Here's how the part is built. I have some questions about the finished solid (model axes, mm). A direction names the side the tool comes from. Give positions to 0.01 mm unless a question says otherwise; leave off trailing zeros. Loops run counter-clockwise (first coordinate to the right, second up) from the corner with the lowest first, then second, coordinate; pieces in that order, holes last. Notation, with made-up numbers: (58, 28.25) -> (108, 28.25) arc R10 ccw to (108, 33.25) -> close; hole circle Ø7 at (-26.5, 80.25). An arc over 180 degrees is marked (long way). Answer in a Markdown table with one row per item. Add a question column.
Item 1: For P1, Ø1.5, axis at y = 25.5, z = -9, coming from the +X side; P2, Ø8, axis at x = -19, z = -1, coming from the +Y side; P3, Ø2.5, axis at x = 20.5, z = 20.5, coming from the +Y side, each with a flat end and sliding along its axis, tell me the tip position at first contact or that it passes through.
Item 2: We'd pull the mould along Z, two halves only. Please class faces 1 (the face through (-27.5, 26, 17)), 2 (the face through (-11.5, 26, 0)): released by +Z, released by -Z, zero draft, split by the parting line, or undercut.
Item 3: Which directions (+Z, -Z, +X, -X, +Y, -Y) give clear straight access to the entire face, cutting with the end or side of a thin tool? Please do faces 3 (the face through (-12, 26, -9)), 4 (the face through (-27.5, 26, -18)), 5 (the face through (-22.5, 25.1, 19.9)), 6 (the face through (27.5, 26, 0)).
Item 4: If I drill on line 1 (Z direction, x = -10, y = 22.75); line 2 (Z direction, x = 8.5, y = 23.5); line 3 (Z direction, x = -20, y = 24), over which ranges is the centre line in solid material (lowest first)?
Item 5: If we section it at A-A (y = 18): Write out the boundary of the cut face in (x, z), then the cut area to 3 significant figures.
Item 6: If we section it at C-C (z = -21): Write out the boundary of the cut face in (x, y).
Item 7: If we section it at D-D (y = 26.5): Give the number of separate pieces and of enclosed holes in the cut face, then the cut area to 3 significant figures.
Item 8: If we section it at B-B (x = -10): Write out the boundary of the cut face in (y, z), then the cut area to 3 significant figures.
Autodesk Inventor part; units mm, degrees
ref_plane "YZ Plane" through (0, 0, 0) normal (1, 0, 0) x (0, 1, 0)
ref_plane "XZ Plane" through (0, 0, 0) normal (0, 1, 0) x (-1, 0, 0)
ref_plane "XY Plane" through (0, 0, 0) normal (0, 0, 1) x (1, 0, 0)
sketch "Sketch1" plane through (0, 0, 0) normal (0, 1, 0) x (-1, 0, 0)
  line L0 (30, 30) -> (-30, 30)
  line L1 (-30, 30) -> (-30, -30)
  line L2 (-30, -30) -> (30, -30)
  line L3 (30, -30) -> (30, 30)
  line L4 (30, 30) -> (-30, -30) construction
  line L5 (-30, 30) -> (30, -30) construction
  point P0 (0, 0)
  dimension "d0" = 60
  dimension "d1" = 60
extrude "Extrusion1" add sketch "Sketch1" along normal blind 22.5
sketch "Sketch2" plane through (0, 22.5, 0) normal (0, 1, 0) x (1, 0, 0)
  line L0 (-27.5, -27.5) -> (27.5, -27.5)
  line L1 (27.5, -27.5) -> (27.5, 27.5)
  line L2 (27.5, 27.5) -> (-27.5, 27.5)
  line L3 (-27.5, 27.5) -> (-27.5, -27.5)
  line L4 (-27.5, -27.5) -> (27.5, 27.5) construction
  line L5 (27.5, -27.5) -> (-27.5, 27.5) construction
  line L6 (30, 30) -> (-30, 30)
  line L7 (-30, 30) -> (-30, -30)
  point P0 (0, 0)
  dimension "d4" = 2.5
  dimension "d5" = 2.5
extrude "Extrusion2" add sketch "Sketch2" along normal blind 7.5
sketch "Sketch5" plane through (0, 30, 0) normal (0, 1, 0) x (1, 0, 0)
  point P0 (0, 0)
sketch "Sketch6" plane through (0, 30, 0) normal (0, 1, 0) x (1, 0, 0)
  circle A0 centre (20, 22.5) radius 2.5
  circle A1 centre (-20, 22.5) radius 2.5
  line L0 (-30, -30) -> (30, -30)
  line L1 (30, -30) -> (30, 30)
  line L2 (-30, 30) -> (-30, -30)
  circle A2 centre (20, -20) radius 2.5
  circle A3 centre (-20, -20) radius 2.5
  line L3 (-27.5, -27.5) -> (27.5, -27.5)
  line L4 (27.5, 27.5) -> (-27.5, 27.5)
  circle A4 centre (-10, -20) radius 2.5
  circle A5 centre (-10, 22.5) radius 2.5
  point P0 (0, 0)
  dimension "d15" = 5
  dimension "d16" = 52.5
  dimension "d17" = 52.5
  dimension "d18" = 10
  dimension "d19" = 10
  dimension "d20" = 5
  dimension "d21" = 5
  dimension "d22" = 10
  dimension "d23" = 10
  dimension "d24" = 10
  dimension "d25" = 10
  dimension "d26" = 5
  dimension "d27" = 55
  dimension "d28" = 57.5
  dimension "d66" = 5
  dimension "d67" = 5
  dimension "d68" = 40
  dimension "d69" = 40
extrude "Extrusion5" cut sketch "Sketch6" against normal blind 10
sketch "Sketch7" plane through (0, 30, 0) normal (0, 1, 0) x (1, 0, 0)
  arc A0 (8.5, -12.5) -> (8.5, 12.5) centre (8.5, 0) ccw
  line L0 (30, -30) -> (30, 30)
  line L1 (8.5, 0) -> (8.5, 12.5)
  line L2 (8.5, 0) -> (8.5, -12.5)
  point P0 (0, 0)
  dimension "d32" = 21.5
extrude "Extrusion6" cut sketch "Sketch7" against normal blind 10
sketch "Sketch8" plane through (0, 30, 0) normal (0, 1, 0) x (1, 0, 0)
  line L0 (-4, -17.5) -> (6, -17.5)
  line L1 (8.5, -15) -> (8.5, 15)
  line L2 (6, 17.5) -> (-4, 17.5)
  line L3 (-6.5, 15) -> (-6.5, -15)
  line L4 (-6.5, -17.5) -> (8.5, 17.5) construction
  line L5 (8.5, -17.5) -> (-6.5, 17.5) construction
  line L6 (30, -30) -> (30, 30)
  line L7 (8.5, -12.5) -> (8.5, 12.5)
  arc A0 (8.5, 12.5) -> (8.5, -12.5) centre (8.5, 0) ccw
  arc A1 (-4, 17.5) -> (-6.5, 15) centre (-4, 15) ccw
  arc A2 (8.5, 15) -> (6, 17.5) centre (6, 15) ccw
  arc A3 (-6.5, -15) -> (-4, -17.5) centre (-4, -15) ccw
  arc A4 (6, -17.5) -> (8.5, -15) centre (6, -15) ccw
  point P0 (0, 0)
  point P1 (1, 0)
  dimension "d35" = 35
  dimension "d37" = 21.5
extrude "Extrusion7" cut sketch "Sketch8" against normal blind 5
sketch "Sketch9" plane through (0, 25, 0) normal (0, 1, 0) x (1, 0, 0)
  line L0 (8.5, -12.5) -> (8.5, 12.5)
  arc A0 (8.5, 12.5) -> (8.5, -12.5) centre (8.5, 0) ccw
  line L1 (8.5, -12.5) -> (8.5, -15)
  line L2 (8.5, 15) -> (8.5, 12.5)
  line L3 (8.5, -12.5) -> (8.5, 12.5)
  point P0 (0, 0)
extrude "Extrusion8" cut sketch "Sketch9" against normal blind 5
sketch "Sketch11" plane through (8.5, 20, 0) normal (0, 1, 0) x (1, 0, 0)
  circle A0 centre (0, 0) radius 2.5
  line L0 (21.5, -30) -> (21.5, 30)
  point P0 (-8.5, 0)
  dimension "d55" = 21.5
  dimension "d56" = 5
extrude "Extrusion10" cut sketch "Sketch11" against normal blind 10
sketch "Sketch12" plane through (0, 30, 0) normal (0, 1, 0) x (1, 0, 0)
  line L0 (-27.5, -27.5) -> (-27.5, 27.5)
  line L1 (-27.5, 0) -> (-19.0189, 0)
  line L2 (-27.5, 10) -> (-27.5, -10)
  line L3 (-11.5, -7.5) -> (-11.5, 7.5)
  line L4 (-14, 10) -> (-27.5, 10)
  line L5 (-14, -10) -> (-27.5, -10)
  line L6 (30, -30) -> (30, 30)
  arc A0 (-11.5, 7.5) -> (-14, 10) centre (-14, 7.5) ccw
  arc A1 (-14, -10) -> (-11.5, -7.5) centre (-14, -7.5) ccw
  point P0 (0, 0)
  dimension "d59" = 20
  dimension "d60" = 10
  dimension "d61" = 41.5
extrude "Extrusion11" cut sketch "Sketch12" against normal blind 7.5
sketch "Sketch13" plane through (0, 30, 0) normal (0, 1, 0) x (1, 0, 0)
  point P0 (0, 0)
sketch "Sketch14" plane through (0, 22.5, 0) normal (0, 1, 0) x (1, 0, 0)
  circle A0 centre (-21.5, 0) radius 5
  line L0 (30, -30) -> (30, 30)
  point P0 (0, 0)
  dimension "d70" = 10
  dimension "d71" = 51.5
extrude "Extrusion12" cut sketch "Sketch14" against normal blind 10
fillet "Fillet1" radius 2.5 1 edges at (-27.5, 26.25, -27.5)
fillet "Fillet2" radius 2.5 1 edges at (-27.5, 26.25, 27.5)
fillet "Fillet3" radius 2.5 1 edges at (27.5, 26.25, 27.5)
fillet "Fillet4" radius 2.5 1 edges at (27.5, 26.25, -27.5)
properties part number "Exercise1"
Recorded:
| question | item | result |
|---|---|---|
| 1 | P1 | stops at x = 27.5 |
| 1 | P2 | stops at y = 22.5 |
| 1 | P3 | stops at y = 20 |
| 2 | face 1 | zero draft |
| 2 | face 2 | undercut |
| 3 | face 3 | -X, +Y |
| 3 | face 4 | +Z, -Z, -X, +Y |
| 3 | face 5 | +Y |
| 3 | face 6 | +Z, -Z, +X, +Y |
| 4 | line 1 | z = -27.5 to -25, -20 to 17.5, 22.5 to 27.5 |
| 4 | line 2 | z = -27.5 to -12.5, 12.5 to 27.5 |
| 4 | line 3 | z = -27.5 to -25, -20 to -10, 10 to 17.5, 22.5 to 27.5 |
| 5 | outline | (-30, -30) -> (30, -30) -> (30, 30) -> (-30, 30) -> close; hole circle Ø10 at (-21.5, 0); hole circle Ø5 at (8.5, 0) |
| 5 | area | 3,500 mm^2 |
| 6 | outline | (-30, 0) -> (30, 0) -> (30, 22.5) -> (27.5, 22.5) -> (27.5, 30) -> (22, 30) -> (22, 20) -> (18, 20) -> (18, 30) -> (-8, 30) -> (-8, 20) -> (-12, 20) -> (-12, 30) -> (-18, 30) -> (-18, 20) -> (-22, 20) -> (-22, 30) -> (-27.5, 30) -> (-27.5, 22.5) -> (-30, 22.5) -> close |
| 7 | separate pieces | 1 |
| 7 | enclosed holes | 7 |
| 7 | area | 1,820 mm^2 |
| 8 | outline | (0, -30) -> (22.5, -30) -> (22.5, -27.5) -> (30, -27.5) -> (30, -25) -> (20, -25) -> (20, -20) -> (30, -20) -> (30, 17.5) -> (20, 17.5) -> (20, 22.5) -> (30, 22.5) -> (30, 27.5) -> (22.5, 27.5) -> (22.5, 30) -> (0, 30) -> close |
| 8 | area | 1,660 mm^2 |
